from build123d import *

# Parameters (mm, degrees)
ESQUISSE1_W             = 105.4
ESQUISSE1_H             = 169
ESQUISSE1_W_2           = 69.4
ESQUISSE1_H_2           = 133
BOSS_EXTRU_1_DEPTH      = 7
CHANFREIN4_SIZE         = 5
CHANFREIN3_SIZE         = 9
ENL_V_MAT_EXTRU_1_REACH = 101.833
ESQUISSE2_R             = 2.3
ENL_V_START             = -5.4
ESQUISSE5_R             = 3.7
ESQUISSE5_R_2           = 2.3
ENL_V_MAT_EXTRU_4_DEPTH = 5.4
ENL_V_START_2           = -4.3
ESQUISSE4_R             = 41
ENL_V_MAT_EXTRU_3_DEPTH = 4.3


with BuildPart() as part:
    # Esquisse1 → Boss.-Extru.1 (new body)
    with BuildSketch(Plane.XY):
        Rectangle(ESQUISSE1_W, ESQUISSE1_H)
        Rectangle(ESQUISSE1_W_2, ESQUISSE1_H_2, mode=Mode.SUBTRACT)
    extrude(amount=-BOSS_EXTRU_1_DEPTH)

    # Chanfrein4
    chanfrein4_edges = [part.edges().sort_by_distance(p)[0] for p in [
        (-52.7, 84.5, -3.5),
        (52.7, 84.5, -3.5),
        (52.7, -84.5, -3.5),
        (-52.7, -84.5, -3.5),
    ]]
    chamfer(chanfrein4_edges, length=CHANFREIN4_SIZE)

    # Chanfrein3
    # the kernel refuses this chamfer: 9 mm, written as the material it takes off along each edge
    with BuildSketch(Plane(origin=(-34.7, -66.5, -7), x_dir=(-0.9996219169112966, 0, -0.0274958766105864), z_dir=(0, 1, 0)), Plane(origin=(34.7, 66.5, -7), x_dir=(0.9996219169112966, 0, -0.0274958766105864), z_dir=(0, -1, 0))) as chanfrein3_piece_1:
        Polygon((CHANFREIN3_SIZE * 0.999621916911, CHANFREIN3_SIZE * 0.0274958766106), (-CHANFREIN3_SIZE * 0.0274958766106, CHANFREIN3_SIZE * 0.999621916911), (0, 0), align=None)
    extrude(amount=133, mode=Mode.SUBTRACT)
    with BuildSketch(Plane(origin=(-34.7, 66.5, -7), x_dir=(0, 0.9996219169112966, -0.02749587661058638), z_dir=(1, 0, 0)), Plane(origin=(34.7, -66.5, -7), x_dir=(0, -0.9996219169112966, -0.02749587661058638), z_dir=(-1, 0, 0))) as chanfrein3_piece_2:
        Polygon((CHANFREIN3_SIZE * 0.999621916911, CHANFREIN3_SIZE * 0.0274958766106), (-CHANFREIN3_SIZE * 0.0274958766106, CHANFREIN3_SIZE * 0.999621916911), (0, 0), align=None)
    extrude(amount=69.4, mode=Mode.SUBTRACT)
    with BuildSketch(Plane(origin=(-34.7, -89.645146892, -7), x_dir=(-0.9996219169112966, 0, -0.0274958766105864), z_dir=(0, 1, 0))) as chanfrein3_piece_3a_section:
        Polygon((CHANFREIN3_SIZE * 0.999621916911, CHANFREIN3_SIZE * 0.0274958766106), (-CHANFREIN3_SIZE * 0.0274958766106, CHANFREIN3_SIZE * 0.999621916911), (0, 0), align=None)
    chanfrein3_piece_3a = extrude(amount=156.145146892, mode=Mode.PRIVATE)
    chanfrein3_piece_3a = split(chanfrein3_piece_3a, bisect_by=Plane(origin=(-37.668142641, -66.5, -4.031857359), z_dir=(0, -1, 0)), keep=Keep.TOP, mode=Mode.PRIVATE)
    with BuildSketch(Plane(origin=(34.7, -66.5, -7), x_dir=(0, -0.9996219169112966, -0.02749587661058638), z_dir=(-1, 0, 0))) as chanfrein3_piece_3b_section:
        Polygon((CHANFREIN3_SIZE * 0.999621916911, CHANFREIN3_SIZE * 0.0274958766106), (-CHANFREIN3_SIZE * 0.0274958766106, CHANFREIN3_SIZE * 0.999621916911), (0, 0), align=None)
    chanfrein3_piece_3b = extrude(amount=92.545146892, mode=Mode.PRIVATE)
    chanfrein3_piece_3b = split(chanfrein3_piece_3b, bisect_by=Plane(origin=(-34.7, -69.468142641, -4.031857359), z_dir=(-1, 0, 0)), keep=Keep.TOP, mode=Mode.PRIVATE)
    chanfrein3_piece_3 = chanfrein3_piece_3a & chanfrein3_piece_3b
    add(chanfrein3_piece_3, mode=Mode.SUBTRACT)
    with BuildSketch(Plane(origin=(-34.7, -66.5, -7), x_dir=(-0.9996219169112966, 0, -0.0274958766105864), z_dir=(0, 1, 0))) as chanfrein3_piece_4a_section:
        Polygon((CHANFREIN3_SIZE * 0.999621916911, CHANFREIN3_SIZE * 0.0274958766106), (-CHANFREIN3_SIZE * 0.0274958766106, CHANFREIN3_SIZE * 0.999621916911), (0, 0), align=None)
    chanfrein3_piece_4a = extrude(amount=156.145146892, mode=Mode.PRIVATE)
    chanfrein3_piece_4a = split(chanfrein3_piece_4a, bisect_by=Plane(origin=(-37.668142641, 66.5, -4.031857359), z_dir=(0, 1, 0)), keep=Keep.TOP, mode=Mode.PRIVATE)
    with BuildSketch(Plane(origin=(-57.845146892, 66.5, -7), x_dir=(0, 0.9996219169112966, -0.02749587661058638), z_dir=(1, 0, 0))) as chanfrein3_piece_4b_section:
        Polygon((CHANFREIN3_SIZE * 0.999621916911, CHANFREIN3_SIZE * 0.0274958766106), (-CHANFREIN3_SIZE * 0.0274958766106, CHANFREIN3_SIZE * 0.999621916911), (0, 0), align=None)
    chanfrein3_piece_4b = extrude(amount=92.545146892, mode=Mode.PRIVATE)
    chanfrein3_piece_4b = split(chanfrein3_piece_4b, bisect_by=Plane(origin=(-34.7, 69.468142641, -4.031857359), z_dir=(-1, 0, 0)), keep=Keep.TOP, mode=Mode.PRIVATE)
    chanfrein3_piece_4 = chanfrein3_piece_4a & chanfrein3_piece_4b
    add(chanfrein3_piece_4, mode=Mode.SUBTRACT)
    with BuildSketch(Plane(origin=(34.7, 89.645146892, -7), x_dir=(0.9996219169112966, 0, -0.0274958766105864), z_dir=(0, -1, 0))) as chanfrein3_piece_5a_section:
        Polygon((CHANFREIN3_SIZE * 0.999621916911, CHANFREIN3_SIZE * 0.0274958766106), (-CHANFREIN3_SIZE * 0.0274958766106, CHANFREIN3_SIZE * 0.999621916911), (0, 0), align=None)
    chanfrein3_piece_5a = extrude(amount=156.145146892, mode=Mode.PRIVATE)
    chanfrein3_piece_5a = split(chanfrein3_piece_5a, bisect_by=Plane(origin=(37.668142641, 66.5, -4.031857359), z_dir=(0, 1, 0)), keep=Keep.TOP, mode=Mode.PRIVATE)
    with BuildSketch(Plane(origin=(-34.7, 66.5, -7), x_dir=(0, 0.9996219169112966, -0.02749587661058638), z_dir=(1, 0, 0))) as chanfrein3_piece_5b_section:
        Polygon((CHANFREIN3_SIZE * 0.999621916911, CHANFREIN3_SIZE * 0.0274958766106), (-CHANFREIN3_SIZE * 0.0274958766106, CHANFREIN3_SIZE * 0.999621916911), (0, 0), align=None)
    chanfrein3_piece_5b = extrude(amount=92.545146892, mode=Mode.PRIVATE)
    chanfrein3_piece_5b = split(chanfrein3_piece_5b, bisect_by=Plane(origin=(34.7, 69.468142641, -4.031857359), z_dir=(1, 0, 0)), keep=Keep.TOP, mode=Mode.PRIVATE)
    chanfrein3_piece_5 = chanfrein3_piece_5a & chanfrein3_piece_5b
    add(chanfrein3_piece_5, mode=Mode.SUBTRACT)
    with BuildSketch(Plane(origin=(57.845146892, -66.5, -7), x_dir=(0, -0.9996219169112966, -0.02749587661058638), z_dir=(-1, 0, 0))) as chanfrein3_piece_6a_section:
        Polygon((CHANFREIN3_SIZE * 0.999621916911, CHANFREIN3_SIZE * 0.0274958766106), (-CHANFREIN3_SIZE * 0.0274958766106, CHANFREIN3_SIZE * 0.999621916911), (0, 0), align=None)
    chanfrein3_piece_6a = extrude(amount=92.545146892, mode=Mode.PRIVATE)
    chanfrein3_piece_6a = split(chanfrein3_piece_6a, bisect_by=Plane(origin=(34.7, -69.468142641, -4.031857359), z_dir=(1, 0, 0)), keep=Keep.TOP, mode=Mode.PRIVATE)
    with BuildSketch(Plane(origin=(34.7, 66.5, -7), x_dir=(0.9996219169112966, 0, -0.0274958766105864), z_dir=(0, -1, 0))) as chanfrein3_piece_6b_section:
        Polygon((CHANFREIN3_SIZE * 0.999621916911, CHANFREIN3_SIZE * 0.0274958766106), (-CHANFREIN3_SIZE * 0.0274958766106, CHANFREIN3_SIZE * 0.999621916911), (0, 0), align=None)
    chanfrein3_piece_6b = extrude(amount=156.145146892, mode=Mode.PRIVATE)
    chanfrein3_piece_6b = split(chanfrein3_piece_6b, bisect_by=Plane(origin=(37.668142641, -66.5, -4.031857359), z_dir=(0, -1, 0)), keep=Keep.TOP, mode=Mode.PRIVATE)
    chanfrein3_piece_6 = chanfrein3_piece_6a & chanfrein3_piece_6b
    add(chanfrein3_piece_6, mode=Mode.SUBTRACT)

    # Esquisse2 → Enlèv. mat.-Extru.1 (cut, up to next)
    with BuildSketch(Plane.XY, mode=Mode.PRIVATE) as enl_v_mat_extru_1_sk1:
        with Locations((-46.7, 78.5)):
            Circle(ESQUISSE2_R)
    enl_v_mat_extru_1_tool1 = extrude(enl_v_mat_extru_1_sk1.sketch, amount=-ENL_V_MAT_EXTRU_1_REACH, mode=Mode.PRIVATE) & part.part
    # Esquisse2 → Enlèv. mat.-Extru.1 (cut, up to next)
    with BuildSketch(Plane.XY, mode=Mode.PRIVATE) as enl_v_mat_extru_1_sk2:
        with Locations((46.7, 78.5)):
            Circle(ESQUISSE2_R)
    enl_v_mat_extru_1_tool2 = extrude(enl_v_mat_extru_1_sk2.sketch, amount=-ENL_V_MAT_EXTRU_1_REACH, mode=Mode.PRIVATE) & part.part
    # Esquisse2 → Enlèv. mat.-Extru.1 (cut, up to next)
    with BuildSketch(Plane.XY, mode=Mode.PRIVATE) as enl_v_mat_extru_1_sk3:
        with Locations((-46.7, -78.5)):
            Circle(ESQUISSE2_R)
    enl_v_mat_extru_1_tool3 = extrude(enl_v_mat_extru_1_sk3.sketch, amount=-ENL_V_MAT_EXTRU_1_REACH, mode=Mode.PRIVATE) & part.part
    # Esquisse2 → Enlèv. mat.-Extru.1 (cut, up to next)
    with BuildSketch(Plane.XY, mode=Mode.PRIVATE) as enl_v_mat_extru_1_sk4:
        with Locations((46.7, -78.5)):
            Circle(ESQUISSE2_R)
    enl_v_mat_extru_1_tool4 = extrude(enl_v_mat_extru_1_sk4.sketch, amount=-ENL_V_MAT_EXTRU_1_REACH, mode=Mode.PRIVATE) & part.part
    add(enl_v_mat_extru_1_tool1.solids().sort_by_distance((-46.7, 78.5, 0))[0], mode=Mode.SUBTRACT)
    add(enl_v_mat_extru_1_tool2.solids().sort_by_distance((46.7, 78.5, 0))[0], mode=Mode.SUBTRACT)
    add(enl_v_mat_extru_1_tool3.solids().sort_by_distance((-46.7, -78.5, 0))[0], mode=Mode.SUBTRACT)
    add(enl_v_mat_extru_1_tool4.solids().sort_by_distance((46.7, -78.5, 0))[0], mode=Mode.SUBTRACT)

    # Esquisse5 → Enlèv. mat.-Extru.4 (cut)
    # profile 1 of 4: a face of its own
    with BuildSketch(Plane(origin=(0, 0, -7), x_dir=(-1, 0, 0), z_dir=(0, 0, -1)).offset(ENL_V_START)):
        with Locations((-46.7, 78.5)):
            Circle(ESQUISSE5_R)
        with Locations(Location((-46.7, 78.5, 0), (0, 0, 180))):
            Circle(ESQUISSE5_R_2, mode=Mode.SUBTRACT)
    # profile 2 of 4: a face of its own
    with BuildSketch(Plane(origin=(0, 0, -7), x_dir=(-1, 0, 0), z_dir=(0, 0, -1)).offset(ENL_V_START)):
        with Locations((46.7, 78.5)):
            Circle(ESQUISSE5_R)
        with Locations(Location((46.7, 78.5, 0), (0, 0, 180))):
            Circle(ESQUISSE5_R_2, mode=Mode.SUBTRACT)
    # profile 3 of 4: a face of its own
    with BuildSketch(Plane(origin=(0, 0, -7), x_dir=(-1, 0, 0), z_dir=(0, 0, -1)).offset(ENL_V_START)):
        with Locations((46.7, -78.5)):
            Circle(ESQUISSE5_R)
        with Locations(Location((46.7, -78.5, 0), (0, 0, 180))):
            Circle(ESQUISSE5_R_2, mode=Mode.SUBTRACT)
    # profile 4 of 4: a face of its own
    with BuildSketch(Plane(origin=(0, 0, -7), x_dir=(-1, 0, 0), z_dir=(0, 0, -1)).offset(ENL_V_START)):
        with Locations((-46.7, -78.5)):
            Circle(ESQUISSE5_R)
        with Locations(Location((-46.7, -78.5, 0), (0, 0, 180))):
            Circle(ESQUISSE5_R_2, mode=Mode.SUBTRACT)
    extrude(amount=ENL_V_MAT_EXTRU_4_DEPTH, mode=Mode.SUBTRACT)

    # Esquisse4 → Enlèv. mat.-Extru.3 (cut)
    with BuildSketch(Plane.XY.offset(ENL_V_START_2)):
        with Locations((0, 23.1)):
            Circle(ESQUISSE4_R)
    extrude(amount=ENL_V_MAT_EXTRU_3_DEPTH, mode=Mode.SUBTRACT)


solid = part.part
Geometry: final body of the model. Coordinates: model frame, mm. A direction names the side the tool comes from. Give positions to 0.01 mm unless a question says otherwise; leave off trailing zeros. Write each loop counter-clockwise with the first axis right and the second up, starting at its lowest first coordinate (ties: lowest second). Pieces come first, ordered by that corner, then holes. Notation, with made-up numbers: M -16.75,-26 L 29.25,-26 A16 cw 29.25,-20 Z; hole C 21.5,-38 d8. An arc over 180 degrees is marked long. Answer in a Markdown table with one row per item. Add a question column.
(1) Section A-A on x = -31. Return loops of the section in (y, z).
(2) First-contact query: pin 1 (2 mm diameter, centred on x = 48, y = 79, fed in from -Z). Flat tip, straight axial feed; report the tip coordinate or a pass-through.
(3) Section B-B on y = 3. Return loops of the section in (x, z).
(4) Ray query, line 1 (X direction, y = 78.5, z = -0.95); line 2 (Y direction, x = 46.7, z = -2.9); line 3 (Y direction, x = 46.7, z = -0.5). Return the intervals inside material, ascending.
(5) Reachability of faces 1 (the flat face through (52.7, -1, -3)), 2 (the flat face through (44, -78, -1.6)), 3 (the cylindrical face through (-41, 23, -2)) from +Z, -Z, +X, -X, +Y, -Y: full face, straight path, thin tool, end or side. Return the list, or none.
(6) Mould query, pull axis X, two halves, no side actions, for faces 4 (the flat face through (-50.2, 82, -3.5)), 5 (the flat face through (-47, 7, -7)), 6 (the cylindrical face through (46.201, -80.745, -0.789)). Classes: +X half, -X half, draft (parallel to the pull), parting line (faces both ways), or undercut.
Result set:
| question | item | result |
|---|---|---|
| 1 | outline | M -84.5,-7 L -75.5,-7 L -68.5,0 L -84.5,0 Z; M 68.5,0 L 75.5,-7 L 84.5,-7 L 84.5,0 Z |
| 2 | pin 1 | stops at z = -1.6 |
| 3 | outline | M -52.7,-7 L -43.7,-7 L -36.7,0 L -52.7,0 Z; M 36.7,0 L 43.7,-7 L 52.7,-7 L 52.7,0 Z |
| 4 | line 1 | x = -52.7 to -49, -44.4 to 44.4, 49 to 52.7 |
| 4 | line 2 | y = -84.5 to -82.2, -74.8 to 74.8, 82.2 to 84.5 |
| 4 | line 3 | y = -84.5 to -80.8, -76.2 to 76.2, 80.8 to 84.5 |
| 5 | face 1 | +Z, -Z, +X, +Y, -Y |
| 5 | face 2 | -Z |
| 5 | face 3 | +Z, -Z |
| 6 | face 4 | -X half |
| 6 | face 5 | draft |
| 6 | face 6 | undercut |
